from build123d import *

# Parameters (mm, degrees)
F0_W     = 123.205647
F0_H     = 90
F1_DEPTH = 50
F2_W     = 97.983871
F2_H     = 59.879035
F3_DEPTH = 25
F4_W     = 37.923388
F4_H     = 26.491936
F5_DEPTH = 25
F6_R     = 5


with BuildPart() as f1:
    # F0 (on Top) → F1 (new body)
    with BuildSketch(Plane.XY):
        with Locations((0.997982, 5.443549)):
            Rectangle(F0_W, F0_H)
    extrude(amount=F1_DEPTH)

    # F2 (on face) → F3 (cut)
    with BuildSketch(Plane.XY.offset(50)):
        with Locations((2.358871, 4.354839)):
            Rectangle(F2_W, F2_H)
    extrude(amount=-F3_DEPTH, mode=Mode.SUBTRACT)

    # F4 (on face) → F5 (join)
    with BuildSketch(Plane.XY.offset(25)):
        with Locations((1.905242, 5.987903)):
            Rectangle(F4_W, F4_H)
    extrude(amount=F5_DEPTH)

    # F6
    f6_edges = [f1.edges().sort_by_distance(p)[0] for p in [
        (-46.633065, 34.294356, 37.5),
        (-46.633065, -25.584679, 37.5),
        (51.350806, -25.584679, 37.5),
        (51.350806, 34.294356, 37.5),
    ]]
    fillet(f6_edges, radius=F6_R)


solid = f1.part
Check sheet for the modelled part. Datum: model origin and axes. Units: mm. A direction names the side the tool comes from. Give positions to 0.01 mm unless a question says otherwise; leave off trailing zeros. Write each loop counter-clockwise with the first axis right and the second up, starting at its lowest first coordinate (ties: lowest second). Pieces come first, ordered by that corner, then holes. Notation, with made-up numbers: M 9.5,24 L 53.5,24 A16 ccw 53.5,53 Z; hole C -14.5,-1.5 d10. An arc over 180 degrees is marked long. Use one line per item in the form item = value.
(1) Section check D-D on y = -22. Record the boundary of the cut face in (x, z).
Answer block:
outline = M -60.6,0 L 62.6,0 L 62.6,50 L 51.15,50 L 51.15,25 L -46.43,25 L -46.43,50 L -60.6,50 Z
(2) Section check A-A on z = 45. Record the boundary of the cut face in (x, y), plus the area to 3 significant figures.
Answer block:
outline = M -60.6,-39.56 L 62.6,-39.56 L 62.6,50.44 L -60.6,50.44 Z; M -17.06,-7.26 L 20.87,-7.26 L 20.87,19.23 L -17.06,19.23 Z; hole M -46.63,-20.58 A5 ccw -41.63,-25.58 L 46.35,-25.58 A5 ccw 51.35,-20.58 L 51.35,29.29 A5 ccw 46.35,34.29 L -41.63,34.29 A5 ccw -46.63,29.29 Z
area = 6,250 mm2
(3) Section check B-B on x = 17. Record the boundary of the cut face in (y, z), plus the area to 3 significant figures.
Answer block:
outline = M -39.56,0 L 50.44,0 L 50.44,50 L 34.29,50 L 34.29,25 L 19.23,25 L 19.23,50 L -7.26,50 L -7.26,25 L -25.58,25 L -25.58,50 L -39.56,50 Z
area = 3,670 mm2
(4) Draft check along X on faces 1 (the flat face through (51.351, 4, 38)), 2 (the flat face through (2, -7.258, 37)), 3 (the flat face through (0, 36, 50)), 4 (the flat face through (-60.605, 5, 25)). Enter one of: pulls with the +X half, pulls with the -X half, needs draft (parallel to the pull), parting line crosses it, or undercut.
Answer block:
face_1 = undercut
face_2 = undercut
face_3 = needs draft
face_4 = pulls with the -X half
(5) Material ranges on line 1 along X through (y, z) = (6.5, 39); line 2 along Y through (x, z) = (-41, 25.5); line 3 along Z through (x, y) = (18, 31.5), recorded low to high.
Answer block:
line_1 = -60.6 to -46.63, -17.06 to 20.87, 51.35 to 62.6
line_2 = -39.56 to -25.58, 34.29 to 50.44
line_3 = 0 to 25
(6) Section check C-C on y = 22.5. Record the boundary of the cut face in (x, z).
Answer block:
outline = M -60.6,0 L 62.6,0 L 62.6,50 L 51.35,50 L 51.35,25 L -46.63,25 L -46.63,50 L -60.6,50 Z
(7) Depth check by flat-ended pin: P1, Ø4, axis at x = 39.5, y = 19, coming from the +Z side; P2, Ø2, axis at x = 17.5, y = 1, coming from the -Z side. Enter the tip coordinate at first touch or a pass-through.
Answer block:
P1 = 25
P2 = 0
(8) Tool access check on faces 5 (the flat face through (2, 6, 50)), 6 (the flat face through (2, 19.234, 37)). Record the directions out of +Z, -Z, +X, -X, +Y, -Y that give a thin tool (end or side, any length) a straight path to the whole face; none if there is none.
Answer block:
face_5 = +Z, +X, -X, +Y, -Y
face_6 = +Z
